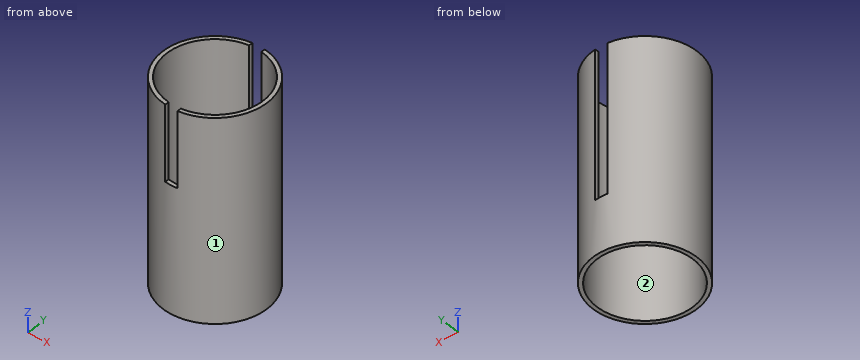
```python
from build123d import *

# Parameters (mm, degrees)
SKETCH1_R           = 41.275
SKETCH1_R_2         = 38.1
BOSS_EXTRUDE1_DEPTH = 160
SKETCH2_W           = 10
SKETCH2_H           = 60
CUT_EXTRUDE1_DEPTH  = 50
SKETCH3_W           = 10
SKETCH3_H           = 117
CUT_EXTRUDE2_DEPTH  = 50


with BuildPart() as part:
    # Sketch1 → Boss-Extrude1 (new body)
    with BuildSketch(Plane.XY):
        Circle(SKETCH1_R)
        Circle(SKETCH1_R_2, mode=Mode.SUBTRACT)
    extrude(amount=BOSS_EXTRUDE1_DEPTH)

    # Sketch2 → Cut-Extrude1 (cut)
    with BuildSketch(Plane(origin=(0, 0, 0), x_dir=(1, 0, 0), z_dir=(0, 1, 0))):
        with Locations((0, -130)):
            Rectangle(SKETCH2_W, SKETCH2_H)
    extrude(amount=-CUT_EXTRUDE1_DEPTH, mode=Mode.SUBTRACT)

    # Sketch3 → Cut-Extrude2 (cut)
    with BuildSketch(Plane(origin=(0, 0, 0), x_dir=(1, 0, 0), z_dir=(0, 1, 0))):
        with Locations((0, -101.5)):
            Rectangle(SKETCH3_W, SKETCH3_H)
    extrude(amount=CUT_EXTRUDE2_DEPTH, mode=Mode.SUBTRACT)


solid = part.part
```
Design review of the part built by this model. Coordinates are the model's own, in mm. Face numbers are marked on the shaded views. Coordinates: 2 decimals unless noted, no trailing zeros. Loops run counter-clockwise (first coordinate to the right, second up) from the corner with the lowest first, then second, coordinate; pieces in that order, holes last.
Q1. We need section A-A on x = 0. State the section outline as (y, z) points (3 decimals).
Reported:
outline: (-41.275, 0) - (-38.1, 0) - (-38.1, 100) - (-41.275, 100) - close; (38.1, 0) - (41.275, 0) - (41.275, 43) - (38.1, 43) - close
Q2. We need section C-C on z = 18.5. State the section outline as (x, y) points (3 decimals).
Reported:
outline: circle Ø82.55 at (0, 0); hole circle Ø76.2 at (0, 0)
Q3. To check wall thickness, follow line 1 (X direction, y = -1, z = 96); line 2 (Y direction, x = 0, z = 55) (3 decimals); line 3 (Y direction, x = 7, z = 115). State the ranges of each line that lie inside material, in increasing order.
Reported:
line 1: x = -41.26 to -38.09, 38.09 to 41.26
line 2: y = -41.275 to -38.1
line 3: y = -40.68 to -37.45, 37.45 to 40.68
Q4. For pin 1 (5 mm diameter, centred on x = -33, z = 29.5, fed in from -Y); pin 2 (6 mm diameter, centred on y = 18, z = 130.5, fed in from -X); pin 3 (2.5 mm diameter, centred on y = 39.5, z = 86, fed in from -X), all flat-tipped, find the tip position at first contact; note any pin that passes through.
Reported:
pin 1: stops at y = -27.81
pin 2: stops at x = -38.45
pin 3: stops at x = -15.51
Q5. The part is to be moulded in two halves that separate along X. For the marked faces 1 and 2, say which applies: +X half, -X half, draft (parallel to the pull), parting line (faces both ways), or undercut.
Reported:
face 1: parting line
face 2: undercut
